Input: part model. Units: mm. Frame: model coordinates. A direction names the side the tool comes from. Give positions to 0.01 mm unless a question says otherwise; leave off trailing zeros. Order: outer loops, then holes, each group sorted by start corner. A loop starts at its lowest first (then second) coordinate and runs counter-clockwise, first axis right, second up. Notation, with made-up numbers: (14.5, 6) - (73.5, 6) arc R30 cw to (73.5, 45) - close; hole circle Ø11 at (70.25, -27). An arc over 180 degrees is marked (long way). Answer in a Markdown table with one row per item. Add a question column.
from build123d import *

# Parameters (mm, degrees)
F1_DEPTH = 7
F6_R     = 5
F6_R_2   = 4.5


with BuildPart() as f1:
    # F0 (on Top) → F1 (new body)
    with BuildSketch(Plane.XY):
        with BuildLine():
            Line((-16.2101432325, 48), (-16.2101432325, 0))
            ThreePointArc((-16.2101432325, 0), (-0.2101432325, -16), (15.7898567675, 0))
            Line((15.7898567675, 0), (15.7898567675, 48))
            ThreePointArc((15.7898567675, 48), (-0.2101432325, 64), (-16.2101432325, 48))
        make_face()
    extrude(amount=F1_DEPTH)

    # F2 (on Right) → F3 (revolve)
    with BuildSketch(Plane.YZ):
        Polygon((33, 97), (19, 97), (19, -105), (24, -105), (24, -90), (31.5, -90), (31.5, 32), (34, 32), (34, 72), (28, 72), (28, 87), (33, 87), align=None)
    revolve(axis=Axis((0, 19, -4), (0, 0, -1)))

    # F7: sweep along a path in F4
    with BuildLine(Plane.YZ) as f7_path:
        Line((-106, 61.7881254457), (-97.95775995, 71.3724939178))
        ThreePointArc((-97.95775995, 71.3724939178), (-90.9776802958, 76.0364340337), (-82.5848076267, 76.2195671668))
        Line((-82.5848076267, 76.2195671668), (19, 49))
    # F6 (on line) → F7 (sweep)
    with BuildSketch(Plane(origin=(0, -13.3719340922, -15.9360504943), x_dir=(1, 0, 0), z_dir=(0, -0.6427876097, -0.7660444431))):
        with Locations((0, 120.9173524329)):
            Circle(F6_R)
        with Locations((0, 120.9173524329)):
            Circle(F6_R_2, mode=Mode.SUBTRACT)
    sweep(path=f7_path.line)


solid = f1.part
Q1. Access query for faces 4 (the cylindrical face through (3.755, 30.923, 19.675)), 5 (the cylindrical face through (-5.362, 31.932, 92.07)), 6 (the cylindrical face through (3.755, 30.923, -44.37)). Directions: +Z, -Z, +X, -X, +Y, -Y. A direction counts if a zero-diameter tool reaches every point of the face in a straight line with its end or side. Return the directions, or none.
Q2. Section A-A, the plane y = 19. Return loops of the section in (x, z).
Q3. Line query: probe 1 along Z at (x, y) = (-10.5, -1); probe 2 along Z at (x, y) = (5.5, 13.5); probe 3 along Z at (x, y) = (1.5, -48). Output: solid intervals per line, ascending.
Q4. Contact query for flat-ended pins moving along their axis: P1, Ø10, axis at x = 12, z = 31.5, coming from the +Y side; P2, Ø12, axis at x = 9.5, z = -76.5, coming from the -Y side; P3, Ø2, axis at x = -12, z = -63.5, coming from the -Y side; P4, Ø8, axis at y = -44.5, z = 54, coming from the -X side. Output: stop coordinate, or through.
Q5. Pull-direction query (Z, two-part tool) for faces 1 (the cylindrical face through (-0.7, -98.1, 63.5)), 2 (the flat face through (-9, 16, 87)), 3 (the cylindrical face through (0, 64, 3)); classes: +Z half, -Z half, draft (parallel to the pull), parting line (faces both ways), or undercut.
Q6. Section B-B, the plane z = -15.5. Return loops of the section in (x, y).
Computed:
| question | item | result |
|---|---|---|
| 1 | face 4 | none |
| 1 | face 5 | +Z |
| 1 | face 6 | -Z |
| 2 | outline | (-16.21, 0) - (-12.5, 0) - (-12.5, -90) - (-5, -90) - (-5, -105) - (5, -105) - (5, -90) - (12.5, -90) - (12.5, 0) - (15.79, 0) - (15.79, 7) - (12.5, 7) - (12.5, 32) - (15, 32) - (15, 72) - (9, 72) - (9, 87) - (14, 87) - (14, 97) - (-14, 97) - (-14, 87) - (-9, 87) - (-9, 72) - (-15, 72) - (-15, 32) - (-12.5, 32) - (-12.5, 7) - (-16.21, 7) - close |
| 3 | probe 1 | z = 0 to 7 |
| 3 | probe 2 | z = -90 to 97 |
| 3 | probe 3 | z = 62.01 to 62.56, 71.34 to 71.89 |
| 4 | P1 | stops at y = 32.25 |
| 4 | P2 | stops at y = 7 |
| 4 | P3 | stops at y = 13.06 |
| 4 | P4 | passes through |
| 5 | face 1 | parting line |
| 5 | face 2 | undercut |
| 5 | face 3 | draft |
| 6 | outline | circle Ø25 at (0, 19) |
